from build123d import *

# Parameters (mm, degrees)
SKETCH_1_R          = 8
EXTRUDE_1_DEPTH     = 6
FILLET_1_R          = 1
SKETCH_3_W          = 3
SKETCH_3_H          = 12
CUT_EXTRUDE_1_DEPTH = 1
FILLET_2_R          = 1
CUT_EXTRUDE_2_DEPTH = 1
CHAMFER_2_SIZE      = 2
CHAMFER_2_SIZE2     = 0.932615316
CHAMFER_5_SIZE      = 2
CHAMFER_5_SIZE2     = 0.848949632
CUT_EXTRUDE_3_DEPTH = 8
CUT_EXTRUDE_START   = -4
SKETCH_7_R          = 7
CUT_EXTRUDE_4_DEPTH = 4


with BuildPart() as part:
    # 草图1 → 凸台-拉伸1 (new body)
    with BuildSketch(Plane(origin=(0, 0, 12), x_dir=(-1, 0, 0), z_dir=(0, 0, -1))):
        Circle(SKETCH_1_R)
    extrude(amount=-EXTRUDE_1_DEPTH)

    # 圆角1
    fillet_1_edges = [part.edges().sort_by_distance(p)[0] for p in [
        (8, 0, 18),
    ]]
    fillet(fillet_1_edges, radius=FILLET_1_R)

    # 草图3 → 切除-拉伸1 (cut)
    with BuildSketch(Plane.XY.offset(18)):
        with Locations((0, -0.105406486)):
            Rectangle(SKETCH_3_W, SKETCH_3_H)
    extrude(amount=-CUT_EXTRUDE_1_DEPTH, mode=Mode.SUBTRACT)

    # 圆角2
    fillet_2_edges = [part.edges().sort_by_distance(p)[0] for p in [
        (-1.5, -6.105406486, 17.5),
        (-1.5, 5.894593514, 17.5),
        (1.5, 5.894593514, 17.5),
        (1.5, -6.105406486, 17.5),
    ]]
    fillet(fillet_2_edges, radius=FILLET_2_R)

    # 草图4 → 切除-拉伸2 (cut)
    with BuildSketch(Plane.XY.offset(18)):
        with BuildLine():
            Line((-6.599663291, 2.333333333), (-4, 2.333333333))
            Line((-4, 2.333333333), (-4, -2.333333333))
            Line((-4, -2.333333333), (-6.599663291, -2.333333333))
            ThreePointArc((-6.599663291, -2.333333333), (-7, 0), (-6.599663291, 2.333333333))
        make_face()
        with BuildLine():
            Line((4, -2.333333333), (6.599663291, -2.333333333))
            ThreePointArc((6.599663291, -2.333333333), (7, 0), (6.599663291, 2.333333333))
            Line((6.599663291, 2.333333333), (4, 2.333333333))
            Line((4, 2.333333333), (4, -2.333333333))
        make_face()
    extrude(amount=-CUT_EXTRUDE_2_DEPTH, mode=Mode.SUBTRACT)

    # 倒角2
    chamfer_2_edges = [part.edges().sort_by_distance(p)[0] for p in [
        (-4, 0, 17),
    ]]
    chamfer_2_side = [part.faces().sort_by_distance(p)[0] for p in [
        (-5.436521823, 0, 17),
    ]]
    chamfer(chamfer_2_edges, length=CHAMFER_2_SIZE, length2=CHAMFER_2_SIZE2, reference=chamfer_2_side[0])

    # 倒角5
    chamfer_5_edges = [part.edges().sort_by_distance(p)[0] for p in [
        (4, 0, 17),
    ]]
    chamfer_5_side = [part.faces().sort_by_distance(p)[0] for p in [
        (5.436521823, 0, 17),
    ]]
    chamfer(chamfer_5_edges, length=CHAMFER_5_SIZE, length2=CHAMFER_5_SIZE2, reference=chamfer_5_side[0])

    # 草图6 → 切除-拉伸3 (cut)
    with BuildSketch(Plane.XY.offset(17)):
        with BuildLine():
            Line((-6.599663291, -2.333333333), (-6, -2.333333333))
            Line((-6, -2.333333333), (-6, 2.333333333))
            Line((-6, 2.333333333), (-6.599663291, 2.333333333))
            ThreePointArc((-6.599663291, 2.333333333), (-7, 0), (-6.599663291, -2.333333333))
        make_face()
        with BuildLine():
            Line((6.599663291, 2.333333333), (6, 2.333333333))
            Line((6, 2.333333333), (6, -2.333333333))
            Line((6, -2.333333333), (6.599663291, -2.333333333))
            ThreePointArc((6.599663291, -2.333333333), (7, 0), (6.599663291, 2.333333333))
        make_face()
    extrude(amount=-CUT_EXTRUDE_3_DEPTH, mode=Mode.SUBTRACT)

    # 草图7 → 切除-拉伸4 (cut)
    with BuildSketch(Plane(origin=(0, 0, 12), x_dir=(-1, 0, 0), z_dir=(0, 0, -1)).offset(CUT_EXTRUDE_START)):
        Circle(SKETCH_7_R)
    extrude(amount=CUT_EXTRUDE_4_DEPTH, mode=Mode.SUBTRACT)


solid = part.part
The listing builds one solid part. Answer for the finished solid, in the listing's coordinates (mm). A direction names the side the tool comes from. Round coordinates to 2 decimals unless told otherwise and drop trailing zeros. Order: outer loops, then holes, each group sorted by start corner. A loop starts at its lowest first (then second) coordinate and runs counter-clockwise, first axis right, second up. Notation, with made-up numbers: M 22.5,-7.5 L 33.5,-7.5 A13 cw 33.5,7.5 Z; hole C -29.5,28 d11. An arc over 180 degrees is marked long. Answer in a Markdown table with one row per item. Add a question column.
1) Consider line 1 along X through (y, z) = (0.25, 17.3); line 2 along Z through (x, y) = (1, -0.5); line 3 along Z through (x, y) = (3.5, -4.5). Determine where each line is inside the solid, lowest interval first. Write a range as from..to.
2) Flat-ended cylindrical pins translate along their axes: pin 1 Ø6.5 at (x, y) = (2, 3) entering from -Z; pin 2 Ø3 at (x, z) = (-4, 15) entering from +Y; pin 3 Ø1.1 at (x, z) = (0, 17.5) entering from +Y; pin 4 Ø2 at (y, z) = (2, 14) entering from +X. Find the tip coordinate at first contact, or state that the pin passes through.
3) Which of the six approach directions +Z, -Z, +X, -X, +Y, -Y give full straight-line access (tool end or side, diameter ignored) to faces 1 (the face through (-4, -6, 12)), 2 (the face through (-6, 0, 16.5)), 3 (the face through (-4.99, 0.03, 17.47))?
4) The part is cut by section B-B on x = 0. Determine the outline of the cut face in (y, z).
5) The part is cut by section A-A on y = 0. Determine the outline of the cut face in (x, z), plus the area to 3 significant figures.
6) Determine the mould class of faces 4 (the face through (6, 0, 16.5)), 5 (the face through (1.73, -7.81, 14.46)), 6 (the face through (2, 0, 18)) for opening direction X: pulls with the +X half, pulls with the -X half, needs draft (parallel to the pull), parting line crosses it, or undercut.
Findings below:
| question | item | result |
|---|---|---|
| 1 | line 1 | x = -7.95..-7, -5.36..-1.5, 1.5..5.29, 7..7.95 |
| 1 | line 2 | z = 16..17 |
| 1 | line 3 | z = 16..18 |
| 2 | pin 1 | stops at z = 16 |
| 2 | pin 2 | stops at y = 7.6 |
| 2 | pin 3 | stops at y = 8 |
| 2 | pin 4 | stops at x = 7.94 |
| 3 | face 1 | -Z, +X, -X, +Y, -Y |
| 3 | face 2 | +Z, -Z |
| 3 | face 3 | +Z |
| 4 | outline | M -8,12 L -7,12 L -7,16 L 7,16 L 7,12 L 8,12 L 8,17 A1 ccw 7,18 L 5.89,18 L 5.89,17 L -6.11,17 L -6.11,18 L -7,18 A1 ccw -8,17 Z |
| 5 | outline | M -8,12 L -7,12 L -7,18 A1 ccw -8,17 Z; M -6,16 L 6,16 L 6,17 L 4,17.85 L 4,18 L 1.5,18 L 1.5,17 L -1.5,17 L -1.5,18 L -4,18 L -4,17.93 L -6,17 Z; M 7,12 L 8,12 L 8,17 A1 ccw 7,18 Z |
| 5 | area | 30.4 mm² |
| 6 | face 4 | undercut |
| 6 | face 5 | parting line crosses it |
| 6 | face 6 | needs draft |
